Part print with two shaded views. Sizes in mm from the minimum x, y, z corner. A direction names the side the tool comes from. Give positions to 0.01 mm unless a question says otherwise; leave off trailing zeros. Write each loop counter-clockwise with the first axis right and the second up, starting at its lowest first coordinate (ties: lowest second). Pieces come first, ordered by that corner, then holes. Notation, with made-up numbers: M -22,-24 L 1,-24 A16 ccw 1,-15 Z; hole C 34,72.25 d6. An arc over 180 degrees is marked long. Return JSON: item names as keys, results as strings. Group by question number.
Q1. Band-saw the part on C-C, the plane z = 7. Give the cut face in (x, y) (1 decimal).
Q2. Band-saw the part on D-D, the plane y = 6.5. Give the cut face in (x, z), then the cut area to 3 significant figures.
Q3. Wall check: probe 1 along Y at (x, z) = (23.25, 3.5); probe 2 along Y at (x, z) = (21.75, 7.5); probe 3 along Y at (x, z) = (4.75, 5.75). Give the ranges that are in metal, low to high.
Q4. Flat gauge pins, fed straight in: pin 1 Ø3 at (x, z) = (3.5, 5.5) entering from -Y; pin 2 Ø3.5 at (x, z) = (23.5, 5) entering from +Y; pin 3 Ø8 at (x, y) = (14.99, 7) entering from +Z; pin 4 Ø2 at (x, z) = (23.5, 3.5) entering from +Y. Where does each tip first touch, or does it go through?
Q5. Band-saw the part on A-A, the plane x = 24. Give the cut face in (y, z).
Q6. Tool access for the marked faces 1, 2, 3, 4 and 5: list every direction of +Z, -Z, +X, -X, +Y, -Y with a clear straight run to the whole face (end or side of a thin tool).
Q7. Pull direction X, two halves, no side cores. Call the marked faces 6, 7 and 8: +X half, -X half, draft (parallel to the pull), parting line (faces both ways), or undercut.
Q8. Band-saw the part on B-B, the plane y = 3. Give the cut face in (x, z).
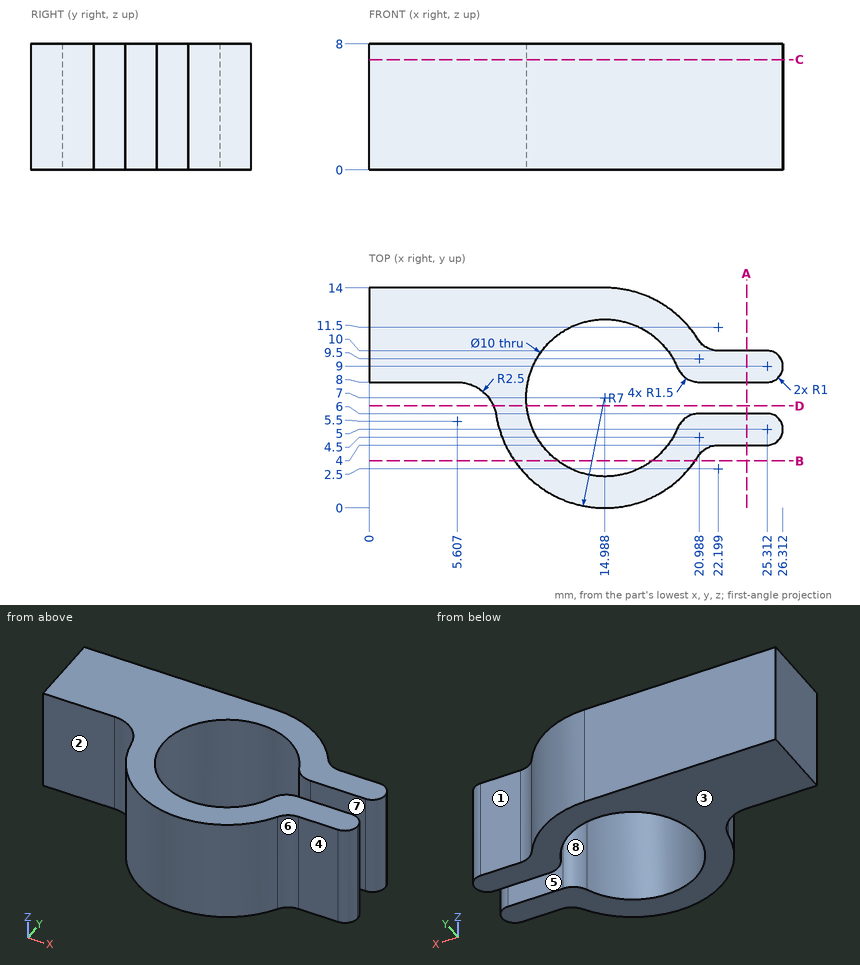
From the geometry:
{
 "1": {"outline": "M 0,8 L 5.6,8 A2.5 cw 8.1,5.9 A7 ccw 20.9,3.3 A1.5 cw 22.2,4 L 25.3,4 A1 ccw 26.3,5 A1 ccw 25.3,6 L 21,6 A1.5 ccw 19.6,5.1 A5 cw long 19.6,8.9 A1.5 ccw 21,8 L 25.3,8 A1 ccw 26.3,9 A1 ccw 25.3,10 L 22.2,10 A1.5 cw 20.9,10.7 A7 ccw 15,14 L 0,14 Z"},
 "2": {"outline": "M 7.9,0 L 10.01,0 L 10.01,8 L 7.9,8 Z", "area": "16.9 mm^2"},
 "3": {"probe 1": "y = 4 to 6, 8 to 10", "probe 2": "y = 3.93 to 6, 8 to 10.07", "probe 3": "y = 8 to 14"},
 "4": {"pin 1": "stops at y = 8", "pin 2": "stops at y = 10.07", "pin 3": "passes through", "pin 4": "stops at y = 10"},
 "5": {"outline": "M 4,0 L 6,0 L 6,8 L 4,8 Z; M 8,0 L 10,0 L 10,8 L 8,8 Z"},
 "6": {"face 1": "+Z, -Z, +X, +Y", "face 2": "+Z, -Z, -X, -Y", "face 3": "-Z, +X, -X, +Y, -Y", "face 4": "+Z, -Z, +X, -Y", "face 5": "+Z, -Z, +X"},
 "7": {"face 6": "+X half", "face 7": "draft", "face 8": "undercut"},
 "8": {"outline": "M 9.24,0 L 11.99,0 L 11.99,8 L 9.24,8 Z; M 17.99,0 L 20.73,0 L 20.73,8 L 17.99,8 Z"}
}
